Source: three-view drawing plus pictorial views. Frame: mm from the lowest corner of the part. Give positions to 0.01 mm unless a question says otherwise; leave off trailing zeros. Loops run counter-clockwise (first coordinate to the right, second up) from the corner with the lowest first, then second, coordinate; pieces in that order, holes last. Notation, with made-up numbers: (54, 55) - (61, 55) arc R12 cw to (61, 71) - close; hole circle Ø5 at (-10, 3.5). An arc over 180 degrees is marked (long way). Answer as a JSON object with one key per item and string values.
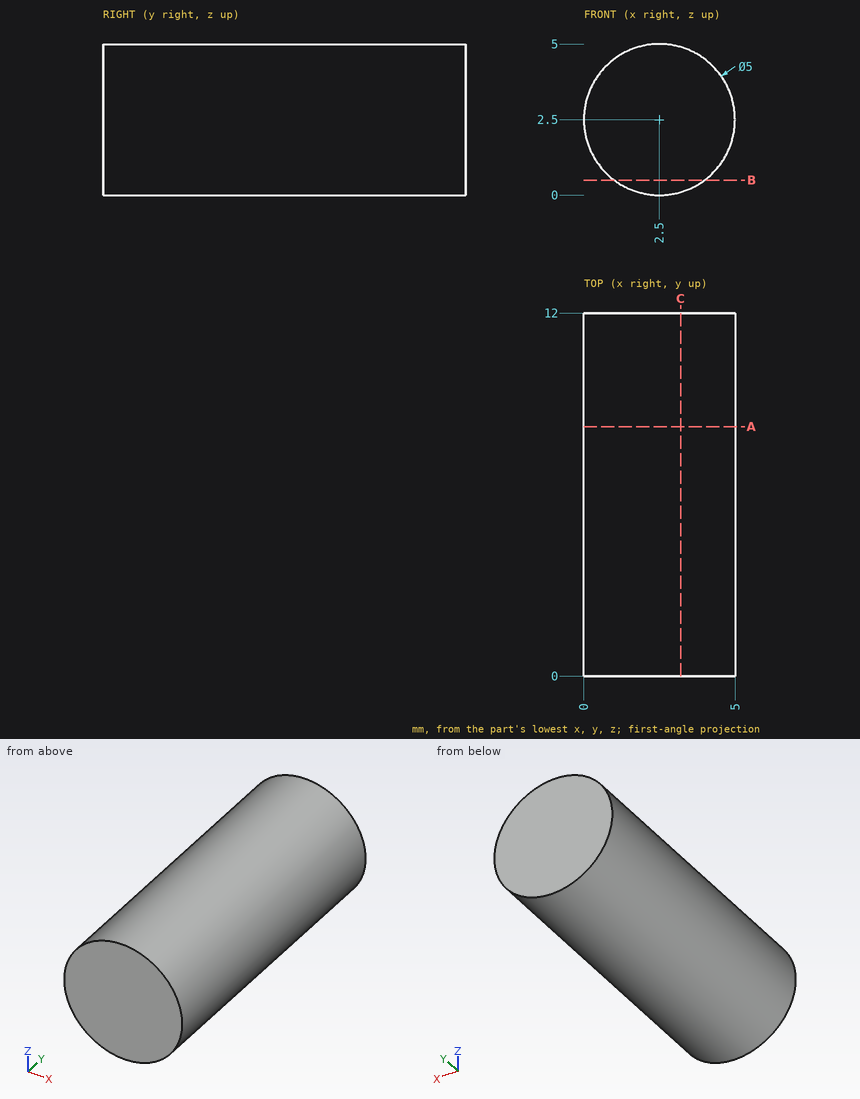
Item 1: Cut plane A-A (y = 8.25). Return loops of the section in (x, z), then the cut area to 3 significant figures.
Geometry check:
{"outline": "circle Ø5 at (2.5, 2.5)", "area": "19.6 mm2"}
Item 2: Cut plane C-C (x = 3.2). Return loops of the section in (y, z).
Geometry check:
{"outline": "(0, 0.1) - (12, 0.1) - (12, 4.9) - (0, 4.9) - close"}
Item 3: Cut plane B-B (z = 0.5). Return loops of the section in (x, y).
Geometry check:
{"outline": "(1, 0) - (4, 0) - (4, 12) - (1, 12) - close"}
Item 4: Contact query for flat-ended pins moving along their axis: P1, Ø2, axis at y = 10.5, z = 1, coming from the -X side; P2, Ø1, axis at x = 1, y = 7.5, coming from the +Z side. Output: stop coordinate, or through.
Geometry check:
{"P1": "stops at x = 0.05", "P2": "stops at z = 4.79"}
Item 5: Material intervals for line 1 (X direction, y = 4.75, z = 4); line 2 (Z direction, x = 0.6, y = 10.5); line 3 (X direction, y = 0.5, z = 3.7), sorted ascending. Write a range as [from, to].
Geometry check:
{"line 1": "x = [0.5, 4.5]", "line 2": "z = [0.88, 4.12]", "line 3": "x = [0.31, 4.69]"}
